Model file for the job. Use its own axes, mm. Round coordinates to 2 decimals unless told otherwise and drop trailing zeros. Order: outer loops, then holes, each group sorted by start corner. A loop starts at its lowest first (then second) coordinate and runs counter-clockwise, first axis right, second up. Notation, with made-up numbers: (20.25, 3.5) - (46.25, 3.5) arc R13 cw to (46.25, 27.5) - close; hole circle Ø4 at (87.5, -34.75). An arc over 180 degrees is marked (long way). Write item = value, one per line.
```python
from build123d import *

# Parameters (mm, degrees)
SKETCH1_R           = 70
SKETCH1_R_2         = 3.175
BOSS_EXTRUDE2_DEPTH = 5
SKETCH2_R           = 5
SKETCH2_R_2         = 3.175
BOSS_EXTRUDE4_DEPTH = 15
SKETCH5_R           = 2
CUT_EXTRUDE4_DEPTH  = 101.124921973


with BuildPart() as part:
    # Sketch1 → Boss-Extrude2 (new body)
    with BuildSketch(Plane(origin=(0, 0, 0), x_dir=(1, 0, 0), z_dir=(0, 1, 0))):
        with Locations(Location((0, 0, 0), (0, 0, 270))):
            Circle(SKETCH1_R)
        with Locations(Location((0, 0, 0), (0, 0, 270))):
            Circle(SKETCH1_R_2, mode=Mode.SUBTRACT)
    extrude(amount=BOSS_EXTRUDE2_DEPTH)

    # Sketch2 → Boss-Extrude4 (add)
    with BuildSketch(Plane(origin=(0, 5, 0), x_dir=(1, 0, 0), z_dir=(0, 1, 0))):
        with Locations(Location((0, 0, 0), (0, 0, 270))):
            Circle(SKETCH2_R)
        with Locations(Location((0, 0, 0), (0, 0, 270))):
            Circle(SKETCH2_R_2, mode=Mode.SUBTRACT)
    extrude(amount=BOSS_EXTRUDE4_DEPTH)

    # Sketch5 → Cut-Extrude4 (cut, through all)
    with BuildSketch(Plane(origin=(0, 5, 0), x_dir=(1, 0, 0), z_dir=(0, 1, 0))):
        with Locations(Location((-61.041759509, 14.033218695, 0), (0, 0, 270))):
            Circle(SKETCH5_R)
        with Locations(Location((-37.041759509, 14.033218695, 0), (0, 0, 270))):
            Circle(SKETCH5_R)
        with Locations(Location((-61.041759509, -13.966781305, 0), (0, 0, 270))):
            Circle(SKETCH5_R)
        with Locations(Location((-37.041759509, -13.966781305, 0), (0, 0, 270))):
            Circle(SKETCH5_R)
        with Locations(Location((37.041759509, 14.033218695, 0), (0, 0, 270))):
            Circle(SKETCH5_R)
        with Locations(Location((61.041759509, 14.033218695, 0), (0, 0, 270))):
            Circle(SKETCH5_R)
        with Locations(Location((37.041759509, -13.966781305, 0), (0, 0, 270))):
            Circle(SKETCH5_R)
        with Locations(Location((61.041759509, -13.966781305, 0), (0, 0, 270))):
            Circle(SKETCH5_R)
    extrude(amount=-CUT_EXTRUDE4_DEPTH, mode=Mode.SUBTRACT)


solid = part.part
```
1) Cut at D-D (z = -49). Write the cut outline in (x, y).
Conclusion:
outline = (-49.99, 0) - (49.99, 0) - (49.99, 5) - (-49.99, 5) - close
2) Cut at C-C (y = 10.75). Write the cut outline in (x, z) (3 decimals).
Conclusion:
outline = circle Ø10 at (0, 0); hole circle Ø6.35 at (0, 0)
3) Cut at A-A (x = 0). Write the cut outline in (y, z) (3 decimals), and give its area (3 significant figures).
Conclusion:
outline = (0, -70) - (5, -70) - (5, -5) - (20, -5) - (20, -3.175) - (0, -3.175) - close; (0, 3.175) - (20, 3.175) - (20, 5) - (5, 5) - (5, 70) - (0, 70) - close
area = 723 mm^2
4) Cut at B-B (z = 0). Write the cut outline in (x, y) (3 decimals).
Conclusion:
outline = (-70, 0) - (-3.175, 0) - (-3.175, 20) - (-5, 20) - (-5, 5) - (-70, 5) - close; (3.175, 0) - (70, 0) - (70, 5) - (5, 5) - (5, 20) - (3.175, 20) - close
5) Flat gauge pins, fed straight in: pin 1 Ø3 at (x, z) = (-5, -40) entering from +Y; pin 2 Ø10 at (y, z) = (5, 1.5) entering from -X; pin 3 Ø10 at (y, z) = (5, -48) entering from +X. Where does each tip first touch, or does it go through?
Conclusion:
pin_1 = 5
pin_2 = -70
pin_3 = 55.24
6) Wall check: line 1 along Y through (x, z) = (19, 50.5); line 2 along X through (y, z) = (3.75, -14); line 3 along X through (y, z) = (1.75, -42.5). Give the ranges that are in metal, low to high.
Conclusion:
line_1 = 0 to 5
line_2 = -68.59 to -63.04, -59.04 to -39.04, -35.04 to 35.04, 39.04 to 59.04, 63.04 to 68.59
line_3 = -55.62 to 55.62
7) Mould opens along X. For faces 1 (the face through (1, 5, 15)), 2 (the face through (-4.88, 12.4, -1.08)), 3 (the face through (59.09, 2.54, -14.47)), 4 (the face through (-59.06, 2.54, 13.71)) say: +X half, -X half, draft (parallel to the pull), parting line (faces both ways), or undercut.
Conclusion:
face_1 = draft
face_2 = parting line
face_3 = undercut
face_4 = undercut
